Build history of the part. All positions in model axes, mm. A direction names the side the tool comes from. Round coordinates to 2 decimals unless told otherwise and drop trailing zeros. Write each loop counter-clockwise with the first axis right and the second up, starting at its lowest first coordinate (ties: lowest second). Pieces come first, ordered by that corner, then holes. Notation, with made-up numbers: (11, 62.25) - (24, 62.25) arc R27 cw to (24, 91.25) - close; hole circle Ø3 at (33.25, 79). An arc over 180 degrees is marked (long way). One line per question, with ' | ' between items.
from build123d import *

# Parameters (mm, degrees)
F0_W      = 120
F0_H      = 100
F1_DEPTH  = 25
F2_W      = 110
F2_H      = 90
F3_DEPTH  = 20
F4_R      = 5
F3_FACE_W = 110
F3_FACE_H = 20
F5_DEPTH  = 10
F6_R      = 4.1325775989
F7_DEPTH  = 10


with BuildPart() as f1:
    # F0 (on Front) → F1 (new body)
    with BuildSketch(Plane.XZ):
        Rectangle(F0_W, F0_H)
    extrude(amount=F1_DEPTH)

    # F2 (on face) → F3 (cut)
    with BuildSketch(Plane.XZ.offset(25)):
        Rectangle(F2_W, F2_H)
    extrude(amount=-F3_DEPTH, mode=Mode.SUBTRACT)

    # F4 (on face) + F3_face (on face) → F5 (cut)
    with BuildSketch(Plane(origin=(0, 0, -50), x_dir=(1, 0, 0), z_dir=(0, 0, -1))):
        with Locations((-50, 12.5)):
            Circle(F4_R)
    with BuildSketch(Plane(origin=(0, -15, -45), x_dir=(1, 0, 0), z_dir=(0, 0, 1))):
        Rectangle(F3_FACE_W, F3_FACE_H)
    extrude(amount=-F5_DEPTH, dir=(0, 0, -1), mode=Mode.SUBTRACT)

    # F6 (on face) → F7 (cut)
    with BuildSketch(Plane.XY.offset(50)):
        with Locations((-50, -12.5)):
            Circle(F6_R)
    extrude(amount=-F7_DEPTH, mode=Mode.SUBTRACT)


solid = f1.part
Q1. Saw through at B-B, the plane z = 22.5. List the corners of the cut face in (x, y), then the cut area to 3 significant figures.
Found:
outline: (-60, -25) - (-55, -25) - (-55, -5) - (55, -5) - (55, -25) - (60, -25) - (60, 0) - (-60, 0) - close | area: 800 mm^2
Q2. Drill centre lines: L1, parallel to X at y = -22, z = 8; L2, parallel to Y at x = -50, z = -46.35; L3, parallel to Z at x = -33, y = -11.75. Where is each one in solid material? Low to high. Write a range as from..to.
Found:
L1: -60..-55, 55..60 | L2: -25..-17.5, -7.5..0 | L3: -50..-45, 45..50
Q3. Saw through at A-A, the plane x = -50. List the corners of the cut face in (y, z), then the cut area to 3 significant figures.
Found:
outline: (-25, -50) - (-17.5, -50) - (-17.5, -45) - (-25, -45) - close; (-25, 45) - (-16.63, 45) - (-16.63, 50) - (-25, 50) - close; (-8.37, 45) - (-5, 45) - (-5, -45) - (-7.5, -45) - (-7.5, -50) - (0, -50) - (0, 50) - (-8.37, 50) - close | area: 609 mm^2
Q4. Which spindle directions (+Z, -Z, +X, -X, +Y, -Y) get a long thin tool onto all of the face, cutting with end or side? Do faces 5 (the flat face through (-55, -15, -1)), 6 (the flat face through (-60, -12, -1)). Say none if no direction does.
Found:
face 5: -Y | face 6: +Z, -Z, -X, +Y, -Y
Q5. Drop a flat-ended pin along its axis: pin 1 (10 mm diameter, centred on x = 23, z = -13.5, fed in from -Y). Give the stop position or say it passes through.
Found:
pin 1: y = -5
Q6. Pull direction Z, two halves, no side cores. Call faces 1 (the flat face through (-1, -12, 50)), 2 (the flat face through (-1, -12, -50)), 3 (the flat face through (-1, -15, -45)), 4 (the cylindrical face through (-53.685, -15.879, -47.535)): +Z half, -Z half, draft (parallel to the pull), parting line (faces both ways), or undercut.
Found:
face 1: +Z half | face 2: -Z half | face 3: undercut | face 4: draft
